```python
from build123d import *

# Parameters (mm, degrees)
SKETCH_1_R          = 13.5
EXTRUDE_1_DEPTH     = 20
SKETCH_2_R          = 1.6
CUT_EXTRUDE_1_DEPTH = 28.649593125
CUT_EXTRUDE_START   = -13.25
SKETCH_3_R          = 13.5
SKETCH_3_R_2        = 4
CUT_EXTRUDE_4_DEPTH = 13.25
SKETCH_4_R          = 5
SKETCH_4_R_2        = 4
EXTRUDE_2_DEPTH     = 1.8
SKETCH_5_R          = 4
SKETCH_5_R_2        = 1.6
CUT_EXTRUDE_6_DEPTH = 3
FILLET_1_R          = 2


with BuildPart() as part:
    # ｽｹｯﾁ1 → ﾎﾞｽ - 押し出し1 (new body)
    with BuildSketch(Plane.XY):
        Circle(SKETCH_1_R)
    extrude(amount=EXTRUDE_1_DEPTH)

    # ｽｹｯﾁ2 → ｶｯﾄ - 押し出し1 (cut, through all)
    with BuildSketch(Plane.XY.offset(20)):
        with Locations((0, 10)):
            Circle(SKETCH_2_R)
        with Locations((8.660254038, -5)):
            Circle(SKETCH_2_R)
        with Locations((-8.660254038, -5)):
            Circle(SKETCH_2_R)
    extrude(amount=-CUT_EXTRUDE_1_DEPTH, mode=Mode.SUBTRACT)

    # ｽｹｯﾁ3 → ｶｯﾄ - 押し出し4 (cut)
    with BuildSketch(Plane.XY.offset(20).offset(CUT_EXTRUDE_START)):
        Circle(SKETCH_3_R)
        Circle(SKETCH_3_R_2, mode=Mode.SUBTRACT)
    extrude(amount=CUT_EXTRUDE_4_DEPTH, mode=Mode.SUBTRACT)

    # ｽｹｯﾁ4 → ﾎﾞｽ - 押し出し2 (add)
    with BuildSketch(Plane.XY.offset(6.75)):
        Circle(SKETCH_4_R)
        Circle(SKETCH_4_R_2, mode=Mode.SUBTRACT)
    extrude(amount=EXTRUDE_2_DEPTH)

    # ｽｹｯﾁ5 → ｶｯﾄ - 押し出し6 (cut)
    # profile 1 of 3: a face of its own
    with BuildSketch(Plane.XY.offset(6.75)):
        with Locations((0, 10)):
            Circle(SKETCH_5_R)
        with Locations((0, 10)):
            Circle(SKETCH_5_R_2, mode=Mode.SUBTRACT)
    # profile 2 of 3: a face of its own
    with BuildSketch(Plane.XY.offset(6.75)):
        with Locations((8.660254038, -5)):
            Circle(SKETCH_5_R)
        with Locations((8.660254038, -5)):
            Circle(SKETCH_5_R_2, mode=Mode.SUBTRACT)
    # profile 3 of 3: a face of its own
    with BuildSketch(Plane.XY.offset(6.75)):
        with Locations((-8.660254038, -5)):
            Circle(SKETCH_5_R)
        with Locations((-8.660254038, -5)):
            Circle(SKETCH_5_R_2, mode=Mode.SUBTRACT)
    extrude(amount=-CUT_EXTRUDE_6_DEPTH, mode=Mode.SUBTRACT)

    # ﾌｨﾚｯﾄ1
    # the kernel refuses this fillet: 2 mm, written as the material it takes off along each edge
    with BuildSketch(Plane(origin=(-10.407876243, -8.598029548, 19.555288564), x_dir=(0.7715815777995733, -0.6361303866349423, 0), z_dir=(0, 0, -1)), Plane(origin=(12.650050133, -4.714470452, 19.555288564), x_dir=(0.1651142860452898, 0.9862744407839807, 0), z_dir=(0, 0, -1)), Plane(origin=(-2.242173889, 13.3125, 19.555288564), x_dir=(-0.9366958638448638, -0.35014405414903826, 0), z_dir=(0, 0, -1))) as fillet_1_piece_1:
        with BuildLine():
            CenterArc((4.742699468, -1.963681118), FILLET_1_R, 79.064257334, 119.641084367)
            ThreePointArc((2.848338702, -2.605083713), (1.759195342, -0.936232133), (0, 0))
            ThreePointArc((0, 0), (2.561057713, 0.245152457), (5.122115425, 0))
        make_face()
    extrude(amount=15.805288564, mode=Mode.SUBTRACT)
    with BuildSketch(Plane(origin=(-12.650050133, -4.714470452, 19.555288564), x_dir=(-0.16511428604529083, 0.9862744407839806, 0), z_dir=(0, 0, -1)), Plane(origin=(10.407876243, -8.598029548, 19.555288564), x_dir=(-0.7715815777995731, -0.6361303866349423, 0), z_dir=(0, 0, -1)), Plane(origin=(2.242173889, 13.3125, 19.555288564), x_dir=(0.9366958638448638, -0.35014405414903793, 0), z_dir=(0, 0, -1))) as fillet_1_piece_2:
        with BuildLine():
            CenterArc((4.742699468, 1.963681118), FILLET_1_R, 161.294658299, 119.641084367)
            ThreePointArc((2.848338702, 2.605083713), (1.759195342, 0.936232133), (0, 0))
            ThreePointArc((0, 0), (2.561057713, -0.245152457), (5.122115425, 0))
        make_face()
    extrude(amount=15.805288564, mode=Mode.SUBTRACT)


solid = part.part
```
Geometry: final body of the model. Coordinates: model frame, mm. A direction names the side the tool comes from. Coordinates: 2 decimals unless noted, no trailing zeros. Order: outer loops, then holes, each group sorted by start corner. A loop starts at its lowest first (then second) coordinate and runs counter-clockwise, first axis right, second up. Notation, with made-up numbers: (-6, 56.25) -> (29, 56.25) arc R20 cw to (29, 93.25) -> close; hole circle Ø5 at (-28.75, 44.5). An arc over 180 degrees is marked (long way). Answer in a Markdown table with one row per item.
Item 1: Contact query for flat-ended pins moving along their axis: P1, Ø1.5, axis at y = -4.5, z = 4, coming from the +X side; P2, Ø5, axis at x = -1, y = 4, coming from the -Z side; P3, Ø2.5, axis at x = 8.66, y = -5, coming from the +Z side; P4, Ø1.5, axis at x = -4, y = -5.5, coming from the +Z side. Output: stop coordinate, or through.
Return value:
| item | result |
|---|---|
| P1 | stops at x = 12.96 |
| P2 | stops at z = 0 |
| P3 | passes through |
| P4 | stops at z = 6.75 |
Item 2: Section D-D on x = 11.25. Output: boundary loops of the cut face in (y, z), plus the area to 3 significant figures.
Return value:
| item | result |
|---|---|
| outline | (-7.46, 0) -> (7.46, 0) -> (7.46, 6.75) -> (-1.7, 6.75) -> (-1.7, 3.75) -> (-7.46, 3.75) -> close |
| area | 83.4 mm² |
Item 3: Section C-C on y = 6.5. Output: boundary loops of the cut face in (x, z), plus the area to 3 significant figures.
Return value:
| item | result |
|---|---|
| outline | (-11.83, 0) -> (11.83, 0) -> (11.83, 6.75) -> (1.94, 6.75) -> (1.94, 3.75) -> (-1.94, 3.75) -> (-1.94, 6.75) -> (-11.83, 6.75) -> close |
| area | 148 mm² |
Item 4: Access query for faces 1 (the cylindrical face through (7.5, -10.1, 5.3)), 2 (the cylindrical face through (-1.08, -4.88, 7.64)), 3 (the flat face through (2, 11, 3.75)), 4 (the cylindrical face through (-7.498, -10.185, 5.271)). Directions: +Z, -Z, +X, -X, +Y, -Y. A direction counts if a zero-diameter tool reaches every point of the face in a straight line with its end or side. Return the directions, or none.
Return value:
| item | result |
|---|---|
| face 1 | +Z, +X |
| face 2 | +Z |
| face 3 | +Z, +Y |
| face 4 | +Z, -X |
Item 5: Section A-A on x = 0. Output: boundary loops of the cut face in (y, z), plus the area to 3 significant figures.
Return value:
| item | result |
|---|---|
| outline | (-13.5, 0) -> (8.4, 0) -> (8.4, 3.75) -> (6, 3.75) -> (6, 6.75) -> (5, 6.75) -> (5, 8.55) -> (4, 8.55) -> (4, 20) -> (-4, 20) -> (-4, 8.55) -> (-5, 8.55) -> (-5, 6.75) -> (-13.5, 6.75) -> close; (11.6, 0) -> (13.5, 0) -> (13.5, 3.75) -> (11.6, 3.75) -> close |
| area | 257 mm² |
Item 6: Section B-B on z = 16.75. Output: boundary loops of the cut face in (x, y).
Return value:
| item | result |
|---|---|
| outline | circle Ø8 at (0, 0) |
Item 7: Draft query along Y for faces 5 (the flat face through (7, -6, 3.75)), 6 (the flat face through (0, 0, 0)), 7 (the cylindrical face through (0, 6, 5)). Return one class per face: released by +Y, released by -Y, zero draft, split by the parting line, or undercut.
Return value:
| item | result |
|---|---|
| face 5 | undercut |
| face 6 | zero draft |
| face 7 | released by +Y |
Item 8: Ray query, L1, parallel to Z at x = 7, y = -10.25; L2, parallel to Z at x = -3.5, y = 3.5; L3, parallel to X at y = 10.75, z = 3.25. Return the intervals inside material, ascending.
Return value:
| item | result |
|---|---|
| L1 | z = 0 to 6.75 |
| L2 | z = 0 to 8.55 |
| L3 | x = -8.17 to -1.41, 1.41 to 8.17 |
